The model under review builds one solid part; all positions refer to its coordinate system, in mm. Face numbers are marked on the shaded views. A direction names the side the tool comes from. Round coordinates to 2 decimals unless told otherwise and drop trailing zeros. Write each loop counter-clockwise with the first axis right and the second up, starting at its lowest first coordinate (ties: lowest second). Pieces come first, ordered by that corner, then holes. Notation, with made-up numbers: (-1, 8.25) -> (46, 8.25) arc R29 ccw to (46, 38.25) -> close; hole circle Ø1 at (31, 0). An arc over 180 degrees is marked (long way). Return JSON: item names as keys, results as strings. Group by question number.
1. Take a section at B-B, the plane z = -95.25. Write out the cut boundary in (x, y), then the cut area to 3 significant figures.
2. For line 1 along Y through (x, z) = (-131, 0); line 2 along X through (y, z) = (8.5, 71); line 3 along X through (y, z) = (61.5, -26.5), list the stretches that pass through material, from the lowest coordinate up. Write a range as from..to.
3. Take a section at C-C, the plane x = -131. Write out the cut boundary in (y, z), then the cut area to 3 significant figures.
4. Tool access review of the marked faces 4, 5 and 6: name each direction out of +Z, -Z, +X, -X, +Y, -Y from which nothing blocks a thin tool from reaching the whole face with its end or side.
5. Mouldability with a two-part tool opening along Y and no side actions: class the marked faces 1, 2 and 3 as pulls with the +Y half, pulls with the -Y half, needs draft (parallel to the pull), parting line crosses it, or undercut.
6. Take a section at D-D, the plane y = -30. Write out the cut boundary in (x, z), then the cut area to 3 significant figures.
7. Take a section at A-A, the plane x = 0. Write out the cut boundary in (y, z), then the cut area to 3 significant figures.
8. Clearance check with flat-ended pins moving along their axes: P1, Ø10, axis at y = -35, z = 8, coming from the -X side; P2, Ø2, axis at x = 91, y = 10.5, coming from the -Z side; P3, Ø10, axis at y = 0, z = -90.91, coming from the +X side; P4, Ø24.5, axis at y = -95.25, z = 0, coming from the -X side. State where each tip first meets the part, or that it passes through.
from build123d import *

# Parameters (mm, degrees)
SKETCH1_R                   = 57.15
BASE_EXTRUDE_DEPTH          = 150
BOSS_EXTRUDE1_DEPTH         = 150
BOSS_EXTRUDE1_DEPTH_BACK    = 150
SKETCH2_R                   = 70
FILLET1_R                   = 20
SKETCH18_R                  = 44.45
CUT_EXTRUDE3_DEPTH          = 351.000000086
CUT_EXTRUDE2_REACH          = 353.73
SKETCH15_R                  = 9.5
CIRPATTERN2_COUNT           = 4
SKETCH22_R                  = 67.5
CUT_EXTRUDE5_DEPTH          = 3.1
F_5_8_CLEARANCE_HOLE1_D     = 16.66748
F_5_8_CLEARANCE_HOLE1_DEPTH = 20.75


with BuildPart() as part:
    # Sketch1 → Base-Extrude (new, symmetric)
    with BuildSketch(Plane(origin=(0, 0, 0), x_dir=(0, 0, -1), z_dir=(1, 0, 0))):
        Circle(SKETCH1_R)
    extrude(amount=BASE_EXTRUDE_DEPTH, both=True)

    # Sketch2 → Boss-Extrude1 (add, two sides: drawn at the far end of the back side and taken through both)
    with BuildSketch(Plane(origin=(0, 0, 0), x_dir=(1, 0, 0), z_dir=(0, 1, 0)).offset(-BOSS_EXTRUDE1_DEPTH_BACK)):
        with Locations(Location((0, 0, 0), (0, 0, 270))):
            Circle(SKETCH2_R)
    extrude(amount=BOSS_EXTRUDE1_DEPTH + BOSS_EXTRUDE1_DEPTH_BACK)

    # Sketch3 → Boss-Revolve1 (revolve)
    with BuildSketch(Plane.XY):
        with BuildLine():
            Line((0, -100), (0, 100))
            ThreePointArc((0, 100), (100, 0), (0, -100))
        make_face()
    revolve(axis=Axis((0, -115.862970753, 0), (0, 1, 0)))

    # Fillet1
    fillet1_edges = [part.edges().sort_by_distance(p)[0] for p in [
        (0, -150, -70),
        (0, 150, -70),
    ]]
    fillet(fillet1_edges, radius=FILLET1_R)

    # Sketch18 → Cut-Extrude3 (cut, through all)
    with BuildSketch(Plane.ZY.offset(150)):
        Circle(SKETCH18_R)
    extrude(amount=-CUT_EXTRUDE3_DEPTH, mode=Mode.SUBTRACT)

    # Sketch13 → Boss-Revolve4 (revolve)
    with BuildSketch(Plane.XY, mode=Mode.PRIVATE) as boss_revolve4_sk:
        Polygon((126.15, 57.15), (126.15, 114.3), (146.9, 114.3), (146.9, 67.5), (150, 67.5), (150, 57.15), align=None)
    boss_revolve4 = revolve(boss_revolve4_sk.sketch.rotate(Axis((0, 0, 0), (1, 0, 0)), 90), axis=Axis((0, 0, 0), (1, 0, 0)))

    # Mirror2: Boss-Revolve4 across plane
    add(boss_revolve4.mirror(Plane(origin=(0, 0, 0), x_dir=(0, 0, 1), z_dir=(1, 0, 0))))

    # Sketch15 → Cut-Extrude2 (cut, up to next)
    with BuildSketch(Plane.ZY.offset(146.9), mode=Mode.PRIVATE) as cut_extrude2_sk1:
        with Locations((0, 95.25)):
            Circle(SKETCH15_R)
    cut_extrude2_tool1 = extrude(cut_extrude2_sk1.sketch, amount=-CUT_EXTRUDE2_REACH, mode=Mode.PRIVATE) & part.part
    cut_extrude2 = cut_extrude2_tool1.solids().sort_by_distance((-146.9, 95.25, 0))[0]
    add(cut_extrude2, mode=Mode.SUBTRACT)

    # CirPattern2: Cut-Extrude2 ×4 about axis
    cirpattern2_axis = Axis((0, 0, 0), (1, 0, 0))
    for i in range(1, CIRPATTERN2_COUNT):
        add(cut_extrude2.rotate(cirpattern2_axis, i * 360 / CIRPATTERN2_COUNT), mode=Mode.SUBTRACT)

    # Sketch22 → Cut-Extrude5 (cut)
    with BuildSketch(Plane(origin=(146.9, 0, 0), x_dir=(0, 0, -1), z_dir=(1, 0, 0))):
        with Locations(Location((0, 0, 0), (0, 0, 180))):
            Circle(SKETCH22_R)
    extrude(amount=CUT_EXTRUDE5_DEPTH, mode=Mode.SUBTRACT)

    # 5/8 Clearance Hole1
    with Locations(Plane(origin=(126.15, -86.94526051, 61.229912904), x_dir=(0, 0, 1), z_dir=(-1, 0, 0))):
        with Locations((-61.229912904, 177.798020209), (29.681467244, 86.94526051), (-61.229912904, -3.966119638), (-152.141293051, 86.94526051)):
            Hole(F_5_8_CLEARANCE_HOLE1_D / 2, depth=F_5_8_CLEARANCE_HOLE1_DEPTH)


solid = part.part
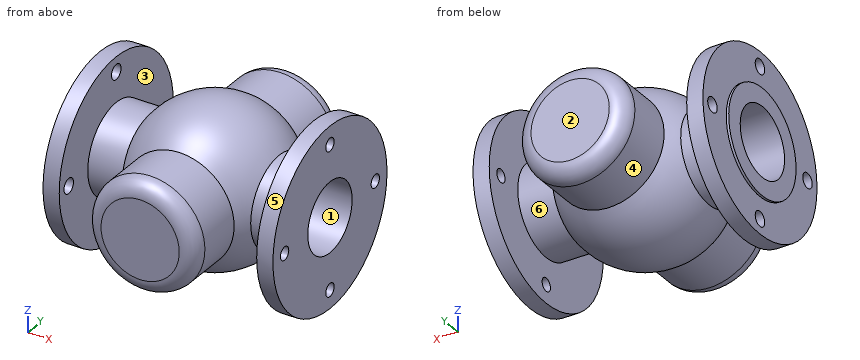
Output:
{
 "1": {"outline": "(-146.9, -63.18) -> (-126.15, -63.18) -> (-126.15, -9.5) -> (-146.9, -9.5) -> close; (-146.9, 9.5) -> (-126.15, 9.5) -> (-126.15, 63.18) -> (-146.9, 63.18) -> close; circle Ø60.91 at (0, 0); (126.15, -63.18) -> (146.9, -63.18) -> (146.9, -7.12) -> (126.15, -7.12) -> close; (126.15, 7.12) -> (146.9, 7.12) -> (146.9, 63.18) -> (126.15, 63.18) -> close", "area": "7,470 mm^2"},
 "2": {"line 1": "y = -114.3..-104.75, -85.75..-44.45, 44.45..85.75, 104.75..114.3", "line 2": "x = -146.9..-126.15, -69.91..69.91, 126.15..146.9", "line 3": "x = -150..-126.15, -74.27..74.27, 126.15..146.9"},
 "3": {"outline": "circle Ø228.6 at (0, 0); hole circle Ø19 at (-95.25, 0); hole circle Ø88.9 at (0, 0); hole circle Ø19 at (0, -95.25); hole circle Ø19 at (0, 95.25); hole circle Ø19 at (95.25, 0)", "area": "33,700 mm^2"},
 "4": {"face 4": "+Y", "face 5": "+X", "face 6": "none"},
 "5": {"face 1": "undercut", "face 2": "pulls with the +Y half", "face 3": "needs draft"},
 "6": {"outline": "(-150, -60.47) -> (-146.9, -60.47) -> (-146.9, -110.29) -> (-126.15, -110.29) -> (-126.15, -48.64) -> (-82.06, -48.64) arc R95.39 ccw to (82.06, -48.64) -> (126.15, -48.64) -> (126.15, -110.29) -> (146.9, -110.29) -> (146.9, -32.8) -> (-150, -32.8) -> close; (-150, 32.8) -> (146.9, 32.8) -> (146.9, 110.29) -> (126.15, 110.29) -> (126.15, 48.64) -> (82.06, 48.64) arc R95.39 ccw to (-82.06, 48.64) -> (-126.15, 48.64) -> (-126.15, 110.29) -> (-146.9, 110.29) -> (-146.9, 60.47) -> (-150, 60.47) -> close", "area": "25,500 mm^2"},
 "7": {"outline": "(-150, -50) arc R20 ccw to (-130, -70) -> (-71.41, -70) arc R100 ccw to (71.41, -70) -> (130, -70) arc R20 ccw to (150, -50) -> (150, 50) arc R20 ccw to (130, 70) -> (71.41, 70) arc R100 ccw to (-71.41, 70) -> (-130, 70) arc R20 ccw to (-150, 50) -> close; hole circle Ø88.9 at (0, 0)", "area": "41,400 mm^2"},
 "8": {"P1": "passes through", "P2": "stops at z = -56.35", "P3": "stops at x = 51.18", "P4": "stops at x = -146.9"}
}
